Source: CAD feature listing. Evaluate the final solid. Frame: model axes, mm. Face numbers are marked on the shaded views. A direction names the side the tool comes from. Round coordinates to 2 decimals unless told otherwise and drop trailing zeros. Loops run counter-clockwise (first coordinate to the right, second up) from the corner with the lowest first, then second, coordinate; pieces in that order, holes last.
(1) Section A-A, the plane z = 12. Return the cut outline in (x, y), plus the area to 3 significant figures.
(2) First-contact query: pin 1 Ø0.7 at (x, z) = (8.5, 13) entering from -Y; pin 2 Ø5 at (x, z) = (-10, 14) entering from -Y; pin 3 Ø8 at (y, z) = (-7.5, 5.5) entering from +X; pin 4 Ø1 at (x, y) = (5, 6) entering from +Z. Flat tips, straight axial feed; report the tip coordinate or a pass-through.
(3) Mould query, pull axis X, two halves, no side actions, for the marked faces 5 and 6. Classes: pulls with the +X half, pulls with the -X half, needs draft (parallel to the pull), parting line crosses it, or undercut.
(4) Section C-C, the plane y = 7.25. Count the separate pieces of the cut face and the enclosed holes in it, plus the area to 3 significant figures.
(5) Material intervals for probe 1 along Y at (x, z) = (0, 2.5); probe 2 along Z at (x, y) = (-8, 7.75); probe 3 along Y at (x, z) = (0, 18.35), sorted ascending.
(6) Set-up query: the marked faces 1, 2, 3 and 4. Return all of +Z, -Z, +X, -X, +Y, -Y with unobstructed straight access to the full face (end or side cutting, diameter ignored); none if empty.
(7) Section D-D, the plane z = 21.3. Return the cut outline in (x, y).
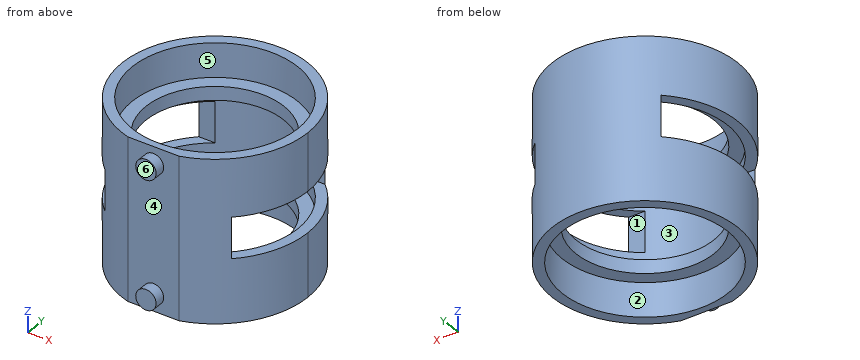
```python
from build123d import *

# Parameters (mm, degrees)
SKETCH1_R               = 12.15
BOSS_EXTRUDE1_DEPTH     = 23.8
BOSS_EXTRUDE2_START     = -7
SKETCH2_R               = 12.15
SKETCH2_R_2             = 10.15
BOSS_EXTRUDE2_DEPTH     = 2
BOSS_EXTRUDE3_START     = -18.8
SKETCH2_2_R             = 12.15
SKETCH2_2_R_2           = 10.15
BOSS_EXTRUDE3_DEPTH     = 2
CUT_EXTRUDE1_DEPTH      = 31.644493796
CUT_EXTRUDE1_DEPTH_BACK = 31.644493796
SKETCH4_W               = 6
SKETCH4_H               = 20
SKETCH5_R               = 1.5
BOSS_EXTRUDE4_DEPTH     = 1.6


with BuildPart() as part:
    # Sketch1 → Boss-Extrude1 (new body)
    with BuildSketch(Plane.XY):
        with BuildLine():
            ThreePointArc((13.65, 0), (-8.213005423, 10.902708009), (-3.766709439, -13.12))
            Line((-3.766709439, -13.12), (3.766709439, -13.12))
            ThreePointArc((3.766709439, -13.12), (10.902708009, -8.213005423), (13.65, 0))
        make_face()
        Circle(SKETCH1_R, mode=Mode.SUBTRACT)
    extrude(amount=BOSS_EXTRUDE1_DEPTH)

    # Sketch2 → Boss-Extrude2 (add)
    with BuildSketch(Plane.XY.offset(23.8).offset(BOSS_EXTRUDE2_START)):
        Circle(SKETCH2_R)
        Circle(SKETCH2_R_2, mode=Mode.SUBTRACT)
    extrude(amount=BOSS_EXTRUDE2_DEPTH)

    # Sketch2_2 → Boss-Extrude3 (add)
    with BuildSketch(Plane.XY.offset(23.8).offset(BOSS_EXTRUDE3_START)):
        Circle(SKETCH2_2_R)
        Circle(SKETCH2_2_R_2, mode=Mode.SUBTRACT)
    extrude(amount=BOSS_EXTRUDE3_DEPTH)

    # Sketch4 → Cut-Extrude1 (cut, two sides: drawn at the far end of the back side and taken through both)
    with BuildSketch(Plane(origin=(0, 0, 0), x_dir=(0, 0, -1), z_dir=(1, 0, 0)).offset(-CUT_EXTRUDE1_DEPTH_BACK)):
        with Locations((-12.335754997, 0)):
            Rectangle(SKETCH4_W, SKETCH4_H)
    extrude(amount=CUT_EXTRUDE1_DEPTH + CUT_EXTRUDE1_DEPTH_BACK, mode=Mode.SUBTRACT)

    # Sketch5 → Boss-Extrude4 (add)
    with BuildSketch(Plane.XZ.offset(13.12)):
        with Locations(Location((0, 21.3, 0), (0, 0, 90))):
            Circle(SKETCH5_R)
        with Locations(Location((0, 2.5, 0), (0, 0, 90))):
            Circle(SKETCH5_R)
    extrude(amount=BOSS_EXTRUDE4_DEPTH)


solid = part.part
```
Output values:
1. outline: (-9.29, -10) arc R13.65 ccw to (-3.77, -13.12) - (3.77, -13.12) arc R13.65 ccw to (9.29, -10) - (6.9, -10) arc R12.15 cw to (-6.9, -10) - close; (-9.29, 10) - (-6.9, 10) arc R12.15 cw to (6.9, 10) - (9.29, 10) arc R13.65 ccw to start
1. area: 50.2 mm2
2. pin 1: stops at y = -10.95
2. pin 2: stops at y = -11.4
2. pin 3: stops at x = 13.19
2. pin 4: passes through
3. face 5: undercut
3. face 6: needs draft
4. separate pieces: 4
4. enclosed holes: 0
4. area: 85.8 mm2
5. probe 1: y = -14.72 to -12.15, 12.15 to 13.65
5. probe 2: z = 5 to 7, 16.8 to 18.8
5. probe 3: y = -13.12 to -10.15, 10.15 to 13.65
6. face 1: +X, -X
6. face 2: -Z
6. face 3: none
6. face 4: -Y
7. outline: (-3.77, -13.12) - (-1.5, -13.12) - (-1.5, -14.72) - (1.5, -14.72) - (1.5, -13.12) - (3.77, -13.12) arc R13.65 ccw (long way) to start; hole circle Ø24.3 at (0, 0)
